Autodesk Inventor part; units mm, degrees
ref_plane "YZ Plane" through (0, 0, 0) normal (1, 0, 0) x (0, 1, 0)
ref_plane "XZ Plane" through (0, 0, 0) normal (0, 1, 0) x (-1, 0, 0)
ref_plane "XY Plane" through (0, 0, 0) normal (0, 0, 1) x (1, 0, 0)
sketch "Sketch1" plane through (0, 0, 0) normal (0, 1, 0) x (-1, 0, 0)
  line L0 (0, 0) -> (0, -29)
  line L1 (0, 0) -> (-25.1147, 14.5)
  line L2 (0, 0) -> (29, 0) construction
  line L3 (0, -29) -> (-3, -29)
  line L4 (-3, -29) -> (-3, -4.2321)
  line L5 (-25.1147, 14.5) -> (-26.6147, 11.9019)
  line L6 (-26.6147, 11.9019) -> (-5.1651, -0.4821)
  arc A0 (-5.1651, -0.4821) -> (-3, -4.2321) centre (-3, -1.7321) ccw
  circle A1 centre (-3, -1.7321) radius 1.5
extrude "Extrusion1" add sketch "Sketch1" along normal blind 24
fillet "Fillet1" radius 1.5 1 edges at (1.5, 24, -29)
fillet "Fillet2" radius 1.5 3 edges at (25.8647, 24, 13.201) (25.8647, 0, 13.201) (1.5, 0, -29)
sketch "Sketch2" plane through (3, 0, -4.2321) normal (1, 0, 0) x (0, 0, -1)
  line L0 (0, 0) -> (23.2679, 0)
  circle A0 centre (20.768, 20) radius 2.5
  circle A1 centre (20.7679, 12) radius 2.5
  circle A2 centre (20.7679, 4) radius 2.5
  line L1 (24.7679, 1.5) -> (24.7679, 22.5)
  circle A3 centre (4.768, 20) radius 2.5
  circle A4 centre (12.768, 20) radius 2.5
  circle A5 centre (12.768, 12) radius 2.5
  circle A6 centre (12.768, 4) radius 2.5
  circle A7 centre (4.768, 4) radius 2.5
  circle A8 centre (4.768, 12) radius 2.5
  point P0 (-4.2321, 0)
sketch "Sketch3" plane through (5.1651, 0, -0.4821) normal (0.5, 0, -0.866) x (-0.866, 0, -0.5)
  circle A0 centre (-20.7679, 20) radius 2.5
  circle A1 centre (-20.7679, 12) radius 2.5
  circle A2 centre (-20.7679, 4) radius 2.5
  circle A3 centre (-12.7679, 4) radius 2.5
  circle A4 centre (-12.7679, 12) radius 2.5
  circle A5 centre (-12.7679, 20) radius 2.5
  circle A6 centre (-4.7679, 20) radius 2.5
  circle A7 centre (-4.7679, 12) radius 2.5
  circle A8 centre (-4.7679, 4) radius 2.5
  point P0 (4.2321, 0)
extrude "Extrusion2" cut sketch "Sketch3" against normal blind 24 contours A2
extrude "Extrusion3" cut sketch "Sketch3" against normal blind 24 contours A0 | A1 | A3 | A4 | A5 | A6 | A7 | A8
extrude "Extrusion4" cut sketch "Sketch2" against normal blind 24
fillet "Fillet3" radius 1.5 1 edges at (0, 12, 0)
properties part number "Bracket Bend 3x3"
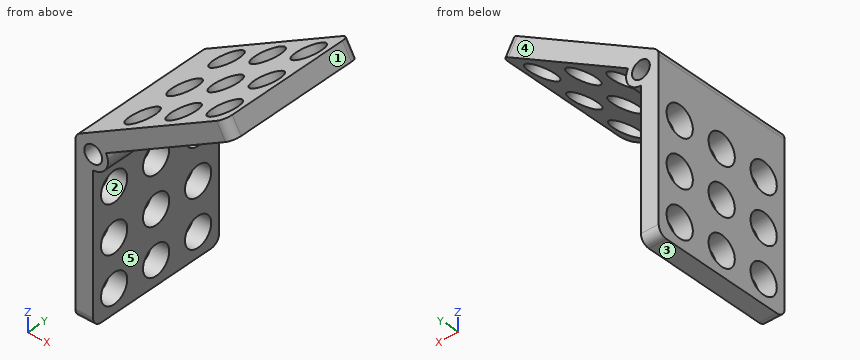
The listing builds one solid part. Answer for the finished solid, in the listing's coordinates (mm). Face numbers are marked on the shaded views. A direction names the side the tool comes from. Give positions to 0.01 mm unless a question says otherwise; leave off trailing zeros. Order: outer loops, then holes, each group sorted by start corner. A loop starts at its lowest first (then second) coordinate and runs counter-clockwise, first axis right, second up.
Item 1: The part is cut by section B-B, the plane z = -17. Give the vertices of the cut face in (x, y).
From the geometry:
outline: (0, 0) - (3, 0) - (3, 1.5) - (0, 1.5) - close; (0, 6.5) - (3, 6.5) - (3, 9.5) - (0, 9.5) - close; (0, 14.5) - (3, 14.5) - (3, 17.5) - (0, 17.5) - close; (0, 22.5) - (3, 22.5) - (3, 24) - (0, 24) - close
Item 2: Given pin 1 Ø5 at (x, y) = (23.5, 18) entering from -Z; pin 2 Ø1.5 at (x, y) = (24, 12) entering from -Z; pin 3 Ø8 at (y, z) = (12, -17) entering from +X, each flat-ended and moving along its own axis, determine where each tip first touches the part or whether it passes through.
From the geometry:
pin 1: stops at z = 8.66
pin 2: stops at z = 12.13
pin 3: stops at x = 3
Item 3: Find the intervals of material crossed by probe 1 along Y at (x, z) = (0.65, -25); probe 2 along X at (y, z) = (16.5, -13.5); probe 3 along Z at (x, y) = (3.5, 1.5), in increasing order.
From the geometry:
probe 1: y = 0 to 1.5, 6.5 to 9.5, 14.5 to 17.5, 22.5 to 24
probe 2: x = 0 to 3
probe 3: z = -4.18 to -3.15, -0.32 to 2.02
Item 4: Which of the six approach directions +Z, -Z, +X, -X, +Y, -Y give full straight-line access (tool end or side, diameter ignored) to the marked faces 4 and 5?
From the geometry:
face 4: +Z, -Z, +X, -X, +Y
face 5: -Z, +X, +Y, -Y
Item 5: The part is cut by section D-D, the plane z = -23. Give the vertices of the cut face in (x, y).
From the geometry:
outline: (0, 0) - (3, 0) - (3, 2.5) - (0, 2.5) - close; (0, 5.5) - (3, 5.5) - (3, 10.5) - (0, 10.5) - close; (0, 13.5) - (3, 13.5) - (3, 18.5) - (0, 18.5) - close; (0, 21.5) - (3, 21.5) - (3, 24) - (0, 24) - close
Item 6: The part is cut by section A-A, the plane y = 13.25. Count the separate pieces of the cut face and the enclosed holes in it, and give its area (3 significant figures).
From the geometry:
separate pieces: 7
enclosed holes: 1
area: 90.2 mm2
Item 7: For a pull along Z with two mould halves and no side action, classify the marked faces 1, 2 and 3 as pulls with the +Z half, pulls with the -Z half, needs draft (parallel to the pull), parting line crosses it, or undercut.
From the geometry:
face 1: pulls with the +Z half
face 2: undercut
face 3: pulls with the -Z half
